Autodesk Inventor part; units mm, degrees
ref_plane "YZ Plane" through (0, 0, 0) normal (1, 0, 0) x (0, 1, 0)
ref_plane "XZ Plane" through (0, 0, 0) normal (0, 1, 0) x (-1, 0, 0)
ref_plane "XY Plane" through (0, 0, 0) normal (0, 0, 1) x (1, 0, 0)
sketch "Náčrt1" plane through (0, 0, 0) normal (0, 0, 1) x (1, 0, 0)
  line L0 (0, 8.68) -> (0, -8.68)
  line L1 (-8.68, 0) -> (8.68, 0)
  circle A0 centre (0, 0) radius 6.2
  dimension "d0" = 12.4
extrude "Vysunutí1" add sketch "Náčrt1" along normal blind 1
sketch "Náčrt2" plane through (0, 0, 1) normal (0, 0, 1) x (1, 0, 0)
  line L0 (-8.68, 0) -> (8.68, 0)
  line L1 (0, 8.68) -> (0, -8.68)
  line L2 (-1.9, 3) -> (1.9, 3)
  line L3 (2.4, 2.5) -> (2.4, -3.5)
  line L4 (1.9, -4) -> (-1.9, -4)
  line L5 (-2.4, -3.5) -> (-2.4, 2.5)
  line L6 (-1.2, 3) -> (1.2, 3)
  line L7 (1.2, 3) -> (1.2, 3.8)
  line L8 (1, 4) -> (-1, 4)
  line L9 (-1.2, 3.8) -> (-1.2, 3)
  arc A0 (-1.9, 3) -> (-2.4, 2.5) centre (-1.9, 2.5) ccw
  arc A1 (2.4, 2.5) -> (1.9, 3) centre (1.9, 2.5) ccw
  arc A2 (-2.4, -3.5) -> (-1.9, -4) centre (-1.9, -3.5) ccw
  arc A3 (1.9, -4) -> (2.4, -3.5) centre (1.9, -3.5) ccw
  arc A4 (-1, 4) -> (-1.2, 3.8) centre (-1, 3.8) ccw
  arc A5 (1.2, 3.8) -> (1, 4) centre (1, 3.8) ccw
  point P0 (0, 0)
  dimension "d3" = 2.4
  dimension "d4" = 2.4
  dimension "d5" = 4
  dimension "d6" = 3
  dimension "d7" = 1.2
  dimension "d8" = 1.2
  dimension "d9" = 1
  dimension "d10" = 0.5
  dimension "d11" = 0.2
extrude "Vysunutí2" add sketch "Náčrt2" along normal blind 0.4
properties part number "button_plate_battery"
Geometry: final body of the model. Coordinates: model frame, mm. A direction names the side the tool comes from. Give positions to 0.01 mm unless a question says otherwise; leave off trailing zeros. Write each loop counter-clockwise with the first axis right and the second up, starting at its lowest first coordinate (ties: lowest second). Pieces come first, ordered by that corner, then holes. Notation, with made-up numbers: (87, 74.5) - (108, 74.5) arc R7 ccw to (108, 83.5) - close; hole circle Ø6 at (33.25, 7.5). An arc over 180 degrees is marked (long way). Return JSON: item names as keys, results as strings. Group by question number.
1) Section A-A on x = 0. Return the cut outline in (y, z).
2) Set-up query: faces 1 (the flat face through (0, 0, 0)), 2 (the flat face through (3, 0, 1)). Return all of +Z, -Z, +X, -X, +Y, -Y with unobstructed straight access to the full face (end or side cutting, diameter ignored); none if empty.
3) Line query: line 1 (Z direction, x = 4.75, y = -0.5); line 2 (X direction, y = -3.25, z = 1.25); line 3 (Y direction, x = 1.5, z = 1.2). Output: solid intervals per line, ascending.
4) Section D-D on y = -5. Return the cut outline in (x, z), plus the area to 3 significant figures.
5) Section B-B on y = 0. Return the cut outline in (x, z).
6) Section C-C on z = 0.6. Return the cut outline in (x, y).
Filled in:
{
 "1": {"outline": "(-6.2, 0) - (6.2, 0) - (6.2, 1) - (4, 1) - (4, 1.4) - (-4, 1.4) - (-4, 1) - (-6.2, 1) - close"},
 "2": {"face 1": "-Z, +X, -X, +Y, -Y", "face 2": "+Z"},
 "3": {"line 1": "z = 0 to 1", "line 2": "x = -2.4 to 2.4", "line 3": "y = -4 to 3"},
 "4": {"outline": "(-3.67, 0) - (3.67, 0) - (3.67, 1) - (-3.67, 1) - close", "area": "7.33 mm^2"},
 "5": {"outline": "(-6.2, 0) - (6.2, 0) - (6.2, 1) - (2.4, 1) - (2.4, 1.4) - (-2.4, 1.4) - (-2.4, 1) - (-6.2, 1) - close"},
 "6": {"outline": "circle Ø12.4 at (0, 0)"}
}
